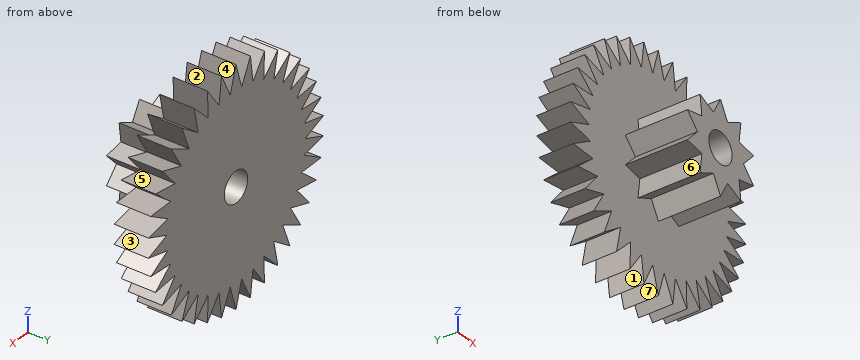
```python
from build123d import *

# Parameters (mm, degrees)
SKETCH2_R          = 0.8
CUT_EXTRUDE1_DEPTH = 6.05
CUT_EXTRUDE2_DEPTH = 6.05
CIRPATTERN1_COUNT  = 38
CUT_EXTRUDE3_DEPTH = 3.25
CIRPATTERN2_COUNT  = 10


with BuildPart() as part:
    # Sketch1 → Revolve1 (revolve)
    with BuildSketch(Plane.XY):
        Polygon((-6.03, 5.05), (-6.03, 3.25), (-2.385, 3.25), (-2.385, 0), (0, 0), (0, 5.05), align=None)
    revolve(axis=Axis((0, 5.05, 0), (0, -1, 0)))

    # Sketch2 → Cut-Extrude1 (cut, through all)
    with BuildSketch(Plane(origin=(0, 5.05, 0), x_dir=(1, 0, 0), z_dir=(0, 1, 0))):
        Circle(SKETCH2_R)
    extrude(amount=-CUT_EXTRUDE1_DEPTH, mode=Mode.SUBTRACT)

    # Sketch3 → Cut-Extrude2 (cut, through all)
    with BuildSketch(Plane(origin=(0, 5.05, 0), x_dir=(1, 0, 0), z_dir=(0, 1, 0))):
        with BuildLine():
            Line((0, 6.03), (0.391691416, 4.727012418))
            Line((0.391691416, 4.727012418), (0.992505379, 5.94775866))
            ThreePointArc((0.992505379, 5.94775866), (0.497953453, 6.009404493), (0, 6.03))
        make_face()
    cut_extrude2 = extrude(amount=-CUT_EXTRUDE2_DEPTH, mode=Mode.SUBTRACT)

    # CirPattern1: Cut-Extrude2 ×38 about axis
    cirpattern1_axis = Axis((0, 0, 0), (0, 1, 0))
    for i in range(1, CIRPATTERN1_COUNT):
        add(cut_extrude2.rotate(cirpattern1_axis, i * 360 / CIRPATTERN1_COUNT), mode=Mode.SUBTRACT)

    # Sketch4 → Cut-Extrude3 (cut)
    with BuildSketch(Plane.XZ):
        with BuildLine():
            Line((1.401867827, 1.929505532), (0.488038951, 1.502029444))
            Line((0.488038951, 1.502029444), (0, 2.385))
            ThreePointArc((0, 2.385), (0.737005532, 2.268269791), (1.401867827, 1.929505532))
        make_face()
    cut_extrude3 = extrude(amount=-CUT_EXTRUDE3_DEPTH, mode=Mode.SUBTRACT)

    # CirPattern2: Cut-Extrude3 ×10 about axis
    cirpattern2_axis = Axis((0, 0, 0), (0, 1, 0))
    for i in range(1, CIRPATTERN2_COUNT):
        add(cut_extrude3.rotate(cirpattern2_axis, i * 360 / CIRPATTERN2_COUNT), mode=Mode.SUBTRACT)


solid = part.part
```
Could you check a few things on this model? Use its own coordinates, in mm. Face numbers are marked on the shaded views. A direction names the side the tool comes from. Give positions to 0.01 mm unless a question says otherwise; leave off trailing zeros. Write each loop counter-clockwise with the first axis right and the second up, starting at its lowest first coordinate (ties: lowest second). Pieces come first, ordered by that corner, then holes. Notation, with made-up numbers: (45, -39) -> (78, -39) arc R35 ccw to (78, -4) -> close; hole circle Ø5 at (60.5, 55). An arc over 180 degrees is marked (long way). Write each question's results on one line, items separated by ' | '.
1. I want a section at A-A, the plane y = 1.25. Write out the boundary of the cut face in (x, z) (1 decimal).
Check sheet entries:
outline: (-2.3, -0.7) -> (-1.3, -0.9) -> (-1.4, -1.9) -> (-0.5, -1.5) -> (0, -2.4) -> (0.5, -1.5) -> (1.4, -1.9) -> (1.3, -0.9) -> (2.3, -0.7) -> (1.6, 0) -> (2.3, 0.7) -> (1.3, 0.9) -> (1.4, 1.9) -> (0.5, 1.5) -> (0, 2.4) -> (-0.5, 1.5) -> (-1.4, 1.9) -> (-1.3, 0.9) -> (-2.3, 0.7) -> (-1.6, 0) -> close; hole circle Ø1.6 at (0, 0)
2. I want a section at B-B, the plane x = 5.25. Write out the boundary of the cut face in (y, z), then the cut area to 3 significant figures.
Check sheet entries:
outline: (3.25, -2.39) -> (5.05, -2.39) -> (5.05, -2.19) -> (3.25, -2.19) -> close; (3.25, -1.51) -> (5.05, -1.51) -> (5.05, -1.12) -> (3.25, -1.12) -> close; (3.25, -0.66) -> (5.05, -0.66) -> (5.05, -0.2) -> (3.25, -0.2) -> close; (3.25, 0.2) -> (5.05, 0.2) -> (5.05, 0.66) -> (3.25, 0.66) -> close; (3.25, 1.12) -> (5.05, 1.12) -> (5.05, 1.51) -> (3.25, 1.51) -> close; (3.25, 2.19) -> (5.05, 2.19) -> (5.05, 2.39) -> (3.25, 2.39) -> close | area: 3.75 mm²
3. I want a section at D-D, the plane z = -1.25. Write out the boundary of the cut face in (x, y).
Check sheet entries:
outline: (-5.46, 3.25) -> (-1.32, 3.25) -> (-1.32, 0) -> (1.32, 0) -> (1.32, 3.25) -> (5.46, 3.25) -> (5.46, 5.05) -> (-5.46, 5.05) -> close
4. I want a section at C-C, the plane z = -5.5. Write out the boundary of the cut face in (x, y), then the cut area to 3 significant figures.
Check sheet entries:
outline: (-1.95, 3.25) -> (-1.81, 3.25) -> (-1.81, 5.05) -> (-1.95, 5.05) -> close; (-1.05, 3.25) -> (-0.77, 3.25) -> (-0.77, 5.05) -> (-1.05, 5.05) -> close; (-0.16, 3.25) -> (0.16, 3.25) -> (0.16, 5.05) -> (-0.16, 5.05) -> close; (0.77, 3.25) -> (1.05, 3.25) -> (1.05, 5.05) -> (0.77, 5.05) -> close; (1.81, 3.25) -> (1.95, 3.25) -> (1.95, 5.05) -> (1.81, 5.05) -> close | area: 2.07 mm²
5. Will these pins go through, and if not, where does the flat tip stop? pin 1 Ø2 at (x, y) = (-2.5, 2.5) entering from -Z; pin 2 Ø3 at (y, z) = (1.5, 0.5) entering from +X.
Check sheet entries:
pin 1: stops at z = -5.7 | pin 2: stops at x = 2.27
6. On a 3-axis mill with a long thin cutter (end or side, diameter ignored), from which of +Z, -Z, +X, -X, +Y, -Y can I reach the whole of each face in a straight line? I mean the marked faces 4, 5, 6 and 7. Say none if no direction works.
Check sheet entries:
face 4: +Z, +Y, -Y | face 5: +Y, -Y | face 6: -X, -Y | face 7: -Z, +Y, -Y
7. I need wall thicknesses on L1, parallel to Y at x = -1, z = 5.25; L2, parallel to X at y = 2.8, z = -2; L3, parallel to X at y = 4.8, z = 1.75. Which ranges of each line are inside material? Lowest first, please.
Check sheet entries:
L1: y = 3.25 to 5.05 | L2: x = -0.21 to 0.21 | L3: x = -4.73 to 4.73
8. If we mould it in two halves opening along Z, with no side actions, what happens to the marked faces 1, 2 and 3? For each: released by +Z, released by -Z, zero draft, split by the parting line, or undercut.
Check sheet entries:
face 1: released by -Z | face 2: released by +Z | face 3: undercut
